Autodesk Inventor part; units mm, degrees
ref_plane "YZ Plane" through (0, 0, 0) normal (1, 0, 0) x (0, 1, 0)
ref_plane "XZ Plane" through (0, 0, 0) normal (0, 1, 0) x (-1, 0, 0)
ref_plane "XY Plane" through (0, 0, 0) normal (0, 0, 1) x (1, 0, 0)
sketch "草圖1" plane through (0, 0, 0) normal (0, 0, 1) x (1, 0, 0)
  line L0 (-56.5, 30) -> (-36.5, 30)
  line L1 (-36.5, 30) -> (-36.5, 0)
  line L2 (-36.5, 0) -> (-56.5, 0)
  line L3 (-56.5, 0) -> (-56.5, 30)
  point P0 (0, 0)
  dimension "d0" = 30
  dimension "d1" = 20
  dimension "d2" = 36.5
extrude "擠出1" add sketch "草圖1" along normal blind 5
sketch "草圖4" plane through (-56.5, 30, 0) normal (0, 1, 0) x (1, 0, 0)
  line L0 (0, 0) -> (58.5, 0)
  line L1 (58.5, 0) -> (58.5, -5)
  line L2 (58.5, -5) -> (0, -5)
  line L3 (0, -5) -> (0, 0)
  line L4 (20, -5) -> (0, -5)
  point P0 (56.5, 0)
  point P1 (18.5, -5)
  point P2 (3, -5)
  dimension "d20" = 5
  dimension "d21" = 0
  dimension "d87" = 58.5
extrude "擠出4" add sketch "草圖4" along normal blind 120
mirror "鏡射1" about plane through (2, 30, 5) normal (1, 0, 0)
sketch "草圖5" plane through (0, 0, 0) normal (0, 0, -1) x (-1, 0, 0)
  line L0 (56.5, 150) -> (-60.5, 150)
  line L1 (-60.5, 150) -> (56.5, 150)
  line L2 (56.5, 150) -> (56.5, 140)
  line L3 (56.5, 140) -> (-60.5, 140)
  line L4 (-60.5, 140) -> (-60.5, 150)
  point P0 (0, 0)
  dimension "d24" = 10
  dimension "d25" = 117
extrude "擠出5" add sketch "草圖5" along normal blind 50
sketch "草圖6" plane through (-56.5, 150, 0) normal (0, 1, 0) x (1, 0, 0)
  line L0 (36, 33.5) -> (73, 33.5)
  line L1 (73, 33.5) -> (73, 41.5)
  line L2 (73, 41.5) -> (36, 41.5)
  line L3 (36, 41.5) -> (36, 33.5)
  line L4 (0, -5) -> (117, -5)
  point P0 (56.5, 0)
  dimension "d28" = 37
  dimension "d29" = 16.5
  dimension "d30" = 8
  dimension "d31" = 38.5
extrude "擠出6" cut sketch "草圖6" against normal up to next
sketch "草圖7" plane through (0, 0, 0) normal (0, 0, -1) x (-1, 0, 0)
  line L0 (56.5, 140) -> (-60.5, 140)
  line L1 (-60.5, 0) -> (-60.5, 140)
  line L2 (-40.5, 0) -> (-60.5, 0)
  line L3 (-40.5, 30) -> (-40.5, 0)
  line L4 (36.5, 30) -> (-40.5, 30)
  line L5 (36.5, 30) -> (36.5, 0)
  line L6 (36.5, 0) -> (56.5, 0)
  line L7 (56.5, 0) -> (56.5, 140)
  point P0 (0, 0)
extrude "擠出7" add sketch "草圖7" along normal blind 5
sketch "草圖11" plane through (0, 0, 5) normal (0, 0, 1) x (1, 0, 0)
  line L0 (-36.5, 86) -> (40.5, 86)
  line L1 (40.5, 86) -> (40.5, 64)
  line L2 (40.5, 64) -> (-36.5, 64)
  line L3 (-36.5, 64) -> (-36.5, 86)
  line L4 (40.5, 0) -> (40.5, 30)
  line L5 (-36.5, 0) -> (-36.5, 30)
  line L6 (40.5, 30) -> (-36.5, 30)
  line L7 (-56.5, 150) -> (60.5, 150)
  point P0 (0, 0)
  dimension "d64" = 0
  dimension "d65" = 0
  dimension "d66" = 34
  dimension "d67" = 64
sketch "草圖12" plane through (0, 0, -5) normal (0, 0, -1) x (-1, 0, 0)
  line L0 (-40.5, 90) -> (36.5, 90)
  line L1 (36.5, 90) -> (36.5, 69)
  line L2 (36.5, 69) -> (-40.5, 69)
  line L3 (-40.5, 69) -> (-40.5, 90)
  line L4 (36.5, 30) -> (36.5, 0)
  line L5 (-40.5, 0) -> (-40.5, 30)
  line L6 (-60.5, 140) -> (56.5, 140)
  line L7 (-40.5, 30) -> (36.5, 30)
  point P0 (0, 0)
  dimension "d68" = 0
  dimension "d69" = 0
  dimension "d70" = 50
  dimension "d71" = 39
loft "斷面混成2" cut profiles "草圖11", "草圖12"
sketch "草圖13" plane through (0, 0, 5) normal (0, 0, 1) x (1, 0, 0)
  circle A0 centre (-45.75, 10.35) radius 1.25
  line L0 (-56.5, 0) -> (-56.5, 150)
  line L1 (-56.5, 0) -> (-36.5, 0)
  circle A1 centre (-45.75, 20.7) radius 1.25
  circle A2 centre (51.25, 10.35) radius 1.25
  circle A3 centre (51.25, 20.7) radius 1.25
  line L2 (40.5, 0) -> (40.5, 30)
  line L3 (60.5, 0) -> (40.5, 0)
  point P0 (0, 0)
  dimension "d76" = 2.5
  dimension "d77" = 10.75
  dimension "d78" = 10.35
  dimension "d79" = 10.35
  dimension "d80" = 10.75
  dimension "d81" = 10.75
  dimension "d82" = 10.75
  dimension "d83" = 10.35
  dimension "d84" = 10.35
extrude "擠出10" cut sketch "草圖13" against normal up to surface (10 mm away)
properties part number "0724"
Can you work these out from the model? Positions are in its coordinate system, mm. A direction names the side the tool comes from. Give positions to 0.01 mm unless a question says otherwise; leave off trailing zeros. Loops run counter-clockwise (first coordinate to the right, second up) from the corner with the lowest first, then second, coordinate; pieces in that order, holes last. Notation, with made-up numbers: M -17.75,68.5 L 18.25,68.5 A23 ccw 18.25,76.5 Z; hole C 27,-38 d10. An arc over 180 degrees is marked long. Use one line per item in the form item = value. Start each with the question number.
(1) On a 3-axis mill with a long thin cutter (end or side, diameter ignored), from which of +Z, -Z, +X, -X, +Y, -Y can I reach the whole of each face in a straight line? I mean faces 1 (the flat face through (3, 88, 0)), 2 (the flat face through (1.461, 66.535, -0.07)), 3 (the flat face through (-2, 145, -33.5)), 4 (the flat face through (3, 102, -5)), 5 (the flat face through (40.5, 15, 0)). Say none if no direction works.
(2) I want a section at A-A, the plane z = -38. Write out the boundary of the cut face in (x, y), and give its area (3 significant figures).
(3) I want a section at C-C, the plane y = 135. Write out the boundary of the cut face in (x, z).
(4) I want a section at B-B, the plane x = 35.5. Write out the boundary of the cut face in (y, z), and give its area (4 significant figures).
(5) I want a section at D-D, the plane z = -22. Write out the boundary of the cut face in (x, y), and give its area (3 significant figures).
(6) I'm going to push flat-ended pins straight in: P1, Ø2, axis at x = 33.5, y = 109.5, coming from the -Z side; P2, Ø6, axis at x = -21.5, y = 69.5, coming from the +Z side; P3, Ø11, axis at x = -7.5, z = 1, coming from the -Y side. Where does each tip first touch, or does it pass through?
(7) Thinking about a two-plate mould opening in X: for faces 6 (the flat face through (-2, 145, -41.5)), 7 (the flat face through (-56.5, 91, -4)), 8 (the flat face through (3, 145, -50)), 9 (the flat face through (60.5, 91, -4)), which applies, released by +X, released by -X, zero draft, split by the parting line, or undercut?
(8) Please list where these lines run through material, in increasing order: line 1 (Y direction, x = -45.75, z = 0.5); line 2 (Y direction, x = -45, z = 3); line 3 (X direction, y = 79, z = 0.5).
Worked out:
q1.face_1 = -Z
q1.face_2 = +Z
q1.face_3 = +Y, -Y
q1.face_4 = -Z, +X, -X, -Y
q1.face_5 = +Z, -Z, -Y
q2.outline = M -56.5,140 L -20.5,140 L -20.5,150 L -56.5,150 Z; M 16.5,140 L 60.5,140 L 60.5,150 L 16.5,150 Z
q2.area = 800 mm²
q3.outline = M -56.5,-5 L 60.5,-5 L 60.5,5 L -56.5,5 Z
q4.outline = M 30,-5 L 69,-5 L 64,5 L 30,5 Z; M 86,5 L 90,-5 L 140,-5 L 140,-50 L 150,-50 L 150,5 Z
q4.area = 1,435 mm²
q5.outline = M -56.5,140 L 60.5,140 L 60.5,150 L -56.5,150 Z
q5.area = 1,170 mm²
q6.P1 = -5
q6.P2 = 0
q6.P3 = 30
q7.face_6 = undercut
q7.face_7 = released by -X
q7.face_8 = zero draft
q7.face_9 = released by +X
q8.line_1 = 0 to 9.1, 11.6 to 19.45, 21.95 to 150
q8.line_2 = 0 to 9.35, 11.35 to 19.7, 21.7 to 150
q8.line_3 = -56.5 to -36.5, 40.5 to 60.5
